Check sheet for the modelled part. Datum: model origin and axes. Units: mm. A direction names the side the tool comes from. Round coordinates to 2 decimals unless told otherwise and drop trailing zeros. Write each loop counter-clockwise with the first axis right and the second up, starting at its lowest first coordinate (ties: lowest second). Pieces come first, ordered by that corner, then holes. Notation, with made-up numbers: (-35.75, 42) - (-9.75, 42) arc R21 cw to (-9.75, 81) - close; hole circle Ø8 at (10, 31.5). An arc over 180 degrees is marked (long way). Answer as a JSON object with one key per item and string values. Group by question number.
Item 1: Sectioned sample at B-B on y = -115. Record the boundary of the cut face in (x, z).
Item 2: Thickness scan on line 1 (Y direction, x = 15, z = -24.5); line 2 (X direction, y = -158, z = 12); line 3 (X direction, y = -160, z = 14.5). Record the ranges inside material, lowest first.
Item 3: Release check for a two-part mould opening along X. For faces 4 (the cylindrical face through (-23, -148.296, 13.775)), 5 (the flat face through (-5.079, -144, 10)), 6 (the flat face through (-21, -109.728, 23)) record: pulls with the +X half, pulls with the -X half, needs draft (parallel to the pull), parting line crosses it, or undercut.
Item 4: Gauge pin test, flat ends, axial feed: P1, Ø11, axis at x = 2, y = -136, coming from the +Z side; P2, Ø9.5, axis at x = 26.5, z = 26, coming from the -Y side; P3, Ø1, axis at x = 20, y = -51, coming from the -Z side; P4, Ø11, axis at y = -153, z = 26, coming from the -X side. Record the tip position at first contact, or that the pin passes through.
Item 5: Sectioned sample at A-A on x = 0. Record the boundary of the cut face in (y, z), plus the area to 3 significant figures.
Item 6: Set-up check for faces 1 (the flat face through (0, -101.295, 18)), 2 (the cylindrical face through (-0.61, -148.3, -20.35)), 3 (the cylindrical face through (23.46, -148.296, 13.484)): record each of +Z, -Z, +X, -X, +Y, -Y from which the full face is reachable in a straight line by a thin tool's end or side.
Item 7: Sectioned sample at D-D on x = -31. Record the boundary of the cut face in (y, z), plus the area to 3 significant figures.
Item 8: Sectioned sample at C-C on z = 15.5. Record the boundary of the cut face in (x, y).
```python
from build123d import *

# Parameters (mm, degrees)
F0_R     = 36.83
F1_DEPTH = 109.728
F3_DEPTH = 78.232
F5_DEPTH = 36.831


with BuildPart() as f1:
    # F0 (on Front) → F1 (new body)
    with BuildSketch(Plane.XZ):
        Circle(F0_R)
    extrude(amount=F1_DEPTH)

    # F2 (on face) → F3 (join)
    with BuildSketch(Plane.XZ.offset(109.728)):
        with BuildLine():
            ThreePointArc((-36.83, 0), (0, -20.352412), (36.83, 0))
            ThreePointArc((36.83, 0), (0, 20.352412), (-36.83, 0))
        make_face()
    extrude(amount=F3_DEPTH)

    # F4 (on Top) → F5 (cut, through all)
    with BuildSketch(Plane.XY):
        Polygon((-5.079485, -101.294816), (-5.079485, -189.798206), (0, -189.798206), (5.079485, -189.798206), (5.079485, -101.294816), align=None)
    extrude(amount=F5_DEPTH, mode=Mode.SUBTRACT)


solid = f1.part
```
Completed:
{
 "1": {"outline": "(-36.83, 0) arc R43.5 ccw to (36.83, 0) arc R43.5 ccw to (5.08, 20.05) - (5.08, 0) - (-5.08, 0) - (-5.08, 20.05) arc R43.5 ccw to start"},
 "2": {"line 1": "-109.73 to 0", "line 2": "-25.63 to -5.08, 5.08 to 25.63", "line 3": "-21.79 to -5.08, 5.08 to 21.79"},
 "3": {"face 4": "pulls with the -X half", "face 5": "undercut", "face 6": "needs draft"},
 "4": {"P1": "z = 20.05", "P2": "y = -109.73", "P3": "z = -31.24", "P4": "through"},
 "5": {"outline": "(-187.96, -20.35) - (-109.73, -20.35) - (-109.73, -36.83) - (0, -36.83) - (0, 36.83) - (-101.29, 36.83) - (-101.29, 0) - (-187.96, 0) - close", "area": "9,360 mm²"},
 "6": {"face 1": "+Z, -Y", "face 2": "-Z, -Y", "face 3": "+Z, +X, -Y"},
 "7": {"outline": "(-187.96, -7.37) - (-109.73, -7.37) - (-109.73, -19.89) - (0, -19.89) - (0, 19.89) - (-109.73, 19.89) - (-109.73, 7.37) - (-187.96, 7.37) - close", "area": "5,520 mm²"},
 "8": {"outline": "(-33.41, -109.73) - (-19.97, -109.73) - (-19.97, -187.96) - (-5.08, -187.96) - (-5.08, -101.29) - (5.08, -101.29) - (5.08, -187.96) - (19.97, -187.96) - (19.97, -109.73) - (33.41, -109.73) - (33.41, 0) - (-33.41, 0) - close"}
}
